Read the model definition and answer for the solid it produces. Units are mm, in the model's axes. A direction names the side the tool comes from. Coordinates: 2 decimals unless noted, no trailing zeros. Write each loop counter-clockwise with the first axis right and the second up, starting at its lowest first coordinate (ties: lowest second). Pieces come first, ordered by that corner, then holes.
(1) Given pin 1 (4 mm diameter, centred on x = 12, y = 10, fed in from +Z); pin 2 (4 mm diameter, centred on x = -19, z = 36.5, fed in from +Y); pin 3 (4 mm diameter, centred on y = 1.5, z = 25.5, fed in from +X); pin 4 (1.5 mm diameter, centred on x = 8, z = 7.5, fed in from -Y), each flat-ended and moving along its own axis, determine where each tip first touches the part or whether it passes through.
(2) Section A-A on x = 0 is taken. Write down the section's boundary in (y, z), then the cut area to 3 significant figures.
(3) Section D-D on z = 30 is taken. Write down the section's boundary in (x, y), then the cut area to 3 significant figures.
(4) Find the intervals of material crossed by probe 1 along X at (y, z) = (0, 28.5); probe 2 along X at (y, z) = (0, 32.5); probe 3 along Y at (x, z) = (0, 30), in increasing order.
(5) Which of the six approach directions +Z, -Z, +X, -X, +Y, -Y give full straight-line access (tool end or side, diameter ignored) to faces 1 (the cylindrical face through (-20.413, 1.146, 39.064)), 2 (the flat face through (18.653, -3.545, 20.28)), 3 (the flat face through (-18.654, -3.545, 20.28)), 4 (the flat face through (1, 13, 40)), 5 (the cylindrical face through (-16.766, -10.297, 4.519))?
(6) Section B-B on z = 37.5 is taken. Write down the section's boundary in (x, y), then the cut area to 3 significant figures.
(7) The mould has two halves that part along Y. Classify faces 6 (the cylindrical face through (-21, -11.43, 1.43)), 7 (the cylindrical face through (2.71, 12.203, 15.585)), 8 (the flat face through (-10.32, -8.02, 15.84)): +Y half, -Y half, draft (parallel to the pull), parting line (faces both ways), or undercut.
(8) Section C-C on z = 4 is taken. State how many separate pieces and enclosed holes the cut face has, then the cut area to 3 significant figures.
from build123d import *

# Parameters (mm, degrees)
EXTRUDE_1_DEPTH     = 40
EXTRUDE_START       = -45.001
EXTRUDE_2_DEPTH     = 45.001
EXTRUDE_2_2_DEPTH   = 41
SKETCH_4_R          = 1.75
CUT_EXTRUDE_1_DEPTH = 51.311943761
CUT_EXTRUDE_2_DEPTH = 7.803062
CUT_EXTRUDE_3_DEPTH = 7.804062
FILLET_6_R          = 5
FILLET_7_R          = 0.5


with BuildPart() as part:
    # ｽｹｯﾁ1 → ﾎﾞｽ - 押し出し1 (new body)
    with BuildSketch(Plane.XY):
        with BuildLine():
            Line((-14.696938457, 3), (-22.5, 3))
            Line((-22.5, 3), (-22.5, 0))
            Line((-22.5, 0), (-12.5, 0))
            ThreePointArc((-12.5, 0), (0, 12.5), (12.5, 0))
            Line((12.5, 0), (22.5, 0))
            Line((22.5, 0), (22.5, 3))
            Line((22.5, 3), (14.696938457, 3))
            ThreePointArc((14.696938457, 3), (0, 15), (-14.696938457, 3))
        make_face()
    extrude(amount=EXTRUDE_1_DEPTH)

    # ﾎﾞｽ - 押し出し2: read off the stored shape, not the designer's step
    # ﾎﾞｽ - 押し出し2 outline → ﾎﾞｽ - 押し出し2 (add)
    with BuildSketch(Plane(origin=(22.5, 0, 0), x_dir=(0, 0, -1), z_dir=(1, 0, 0)).offset(EXTRUDE_START)):
        Polygon((0, -13.276129684), (0, 0), (-40, 0), align=None)
    extrude(amount=EXTRUDE_2_DEPTH)

    # Extrude 2 2 outline → Extrude 2 2 (cut)
    with BuildSketch(Plane.XY):
        with BuildLine():
            ThreePointArc((-12.5, 0), (0, -12.5), (12.5, 0))
            Line((12.5, 0), (-12.5, 0))
        make_face()
    extrude(amount=EXTRUDE_2_2_DEPTH, mode=Mode.SUBTRACT)

    # ｽｹｯﾁ4 → ｶｯﾄ - 押し出し1 (cut, through all)
    with BuildSketch(Plane(origin=(0, -11.958755971, 3.969149878), x_dir=(-1, 0, 0), z_dir=(0, -0.9490896970518627, 0.31500594748354094))):
        with Locations(Location((18.501, -32.963587882, 0), (0, 0, 90))):
            Circle(SKETCH_4_R)
        with Locations(Location((18.501, -0.81794019, 0), (0, 0, 90))):
            Circle(SKETCH_4_R)
        with Locations(Location((-18.5, -32.963587882, 0), (0, 0, 90))):
            Circle(SKETCH_4_R)
        with Locations(Location((-18.5, -0.81794019, 0), (0, 0, 90))):
            Circle(SKETCH_4_R)
    extrude(amount=-CUT_EXTRUDE_1_DEPTH, mode=Mode.SUBTRACT)

    # ｽｹｯﾁ5 → ｶｯﾄ - 押し出し2 (cut)
    with BuildSketch(Plane(origin=(22.5, 0, 0), x_dir=(0, 0, -1), z_dir=(1, 0, 0))):
        Polygon((-40, 3), (0, -10.276129684), (0, 3.043212606), align=None)
    extrude(amount=-CUT_EXTRUDE_2_DEPTH, mode=Mode.SUBTRACT)

    # ｽｹｯﾁ7 → ｶｯﾄ - 押し出し3 (cut)
    with BuildSketch(Plane.ZY.offset(22.501)):
        Polygon((0, 3), (40, 3), (0, -10.276129684), align=None)
    extrude(amount=-CUT_EXTRUDE_3_DEPTH, mode=Mode.SUBTRACT)

    # ﾌｨﾚｯﾄ6
    fillet_6_edges = [part.edges().sort_by_distance(p)[0] for p in [
        (22.5, -11.776129684, 0),
        (22.5, 1.5, 40),
        (-22.5, 1.5, 40),
        (-22.501, -11.776129684, 0),
    ]]
    fillet(fillet_6_edges, radius=FILLET_6_R)

    # ﾌｨﾚｯﾄ7
    fillet_7_edges = [part.edges().sort_by_distance(p)[0] for p in [
        (12.5, 0, 0),
    ]]
    fillet(fillet_7_edges, radius=FILLET_7_R)


solid = part.part
Response:
1. pin 1: stops at z = 40
1. pin 2: stops at y = 2.5
1. pin 3: stops at x = 14.7
1. pin 4: stops at y = -11.04
2. outline: (-13.28, 0) - (-13, 0) arc R0.5 ccw to (-12.5, 0.5) - (-12.5, 2.34) - close; (12.5, 0.5) arc R0.5 ccw to (13, 0) - (15, 0) - (15, 40) - (12.5, 40) - close
2. area: 101 mm2
3. outline: (-22.5, -3.32) - (-12.05, -3.32) arc R12.5 cw (long way) to (12.05, -3.32) - (22.5, -3.32) - (22.5, -0.32) - (14.7, -0.32) - (14.7, 3) arc R15 ccw to (-14.7, 3) - (-14.7, -0.32) - (-22.5, -0.32) - close
3. area: 169 mm2
4. probe 1: x = -14.7 to -12.5, 12.5 to 14.7
4. probe 2: x = -22.5 to -12.5, 12.5 to 22.5
4. probe 3: y = 12.5 to 15
5. face 1: +Z, -X, +Y
5. face 2: -Z, +X, +Y
5. face 3: -Z, -X, +Y
5. face 4: +Z, +X, -X, +Y, -Y
5. face 5: none
6. outline: (-22.5, -0.83) - (-12.47, -0.83) arc R12.5 cw (long way) to (12.47, -0.83) - (21.83, -0.83) - (21.83, 2.17) - (14.7, 2.17) - (14.7, 3) arc R15 ccw to (-14.7, 3) - (-14.7, 2.17) - (-21.83, 2.17) - (-21.83, 0) - (-22.5, 0) - close
6. area: 154 mm2
7. face 6: draft
7. face 7: undercut
7. face 8: -Y half
8. separate pieces: 3
8. enclosed holes: 0
8. area: 241 mm2
